```python
from build123d import *

# Parameters (mm, degrees)
BASE_FLANGE1_DEPTH = 80
CUT_EXTRUDE1_DEPTH = 110.708705215
SKETCH8_R          = 3.5
SKETCH8_W          = 7
SKETCH8_H          = 60
CUT_EXTRUDE2_DEPTH = 111.072703247
CHAMFER1_SIZE      = 2


# Sheet-metal steps are written as plain solids
with BuildPart() as part:
    # Sketch1 → Base-Flange1 (new, symmetric)
    with BuildSketch(Plane(origin=(0, 0, 0), x_dir=(0, 0, -1), z_dir=(1, 0, 0))):
        with BuildLine():
            Line((0, 50), (0, 8))
            ThreePointArc((0, 8), (2.343145751, 2.343145751), (8, 0))
            Line((8, 0), (60, 0))
            Line((60, 0), (60, 4))
            Line((60, 4), (8, 4))
            ThreePointArc((8, 4), (5.171572875, 5.171572875), (4, 8))
            Line((4, 8), (4, 50))
            Line((4, 50), (0, 50))
        make_face()
    extrude(amount=BASE_FLANGE1_DEPTH, both=True)

    # Sketch7 → Cut-Extrude1 (cut, through all)
    with BuildSketch(Plane(origin=(0, 0, -4), x_dir=(-1, 0, 0), z_dir=(0, 0, -1))):
        with BuildLine():
            Line((2.75, 50), (-2.75, 50))
            Line((-2.75, 50), (-2.75, 25))
            ThreePointArc((-2.75, 25), (0, 27.75), (2.75, 25))
            Line((2.75, 25), (2.75, 50))
        make_face()
        with BuildLine():
            ThreePointArc((2.75, 25), (0, 27.75), (-2.75, 25))
            Line((-2.75, 25), (2.75, 25))
        make_face()
        with BuildLine():
            Line((2.75, 25), (-2.75, 25))
            ThreePointArc((-2.75, 25), (0, 22.25), (2.75, 25))
        make_face()
        Polygon((-80, 30), (-25, 50), (-80, 50), align=None)
        Polygon((80, 50), (25, 50), (80, 30), align=None)
    extrude(amount=-CUT_EXTRUDE1_DEPTH, mode=Mode.SUBTRACT)

    # Sketch8 → Cut-Extrude2 (cut, through all)
    with BuildSketch(Plane(origin=(0, 4, 0), x_dir=(1, 0, 0), z_dir=(0, 1, 0))):
        with Locations((-55, 30)):
            Circle(SKETCH8_R)
        with Locations((55, 30)):
            Circle(SKETCH8_R)
        with Locations((-55, 60)):
            Rectangle(SKETCH8_W, SKETCH8_H)
        with Locations((55, 60)):
            Rectangle(SKETCH8_W, SKETCH8_H)
    extrude(amount=-CUT_EXTRUDE2_DEPTH, mode=Mode.SUBTRACT)

    # Chamfer1
    chamfer1_edges = [part.edges().sort_by_distance(p)[0] for p in [
        (80, 2, -60),
        (-80, 2, -60),
    ]]
    chamfer(chamfer1_edges, length=CHAMFER1_SIZE)


solid = part.part
```
Can you work these out from the model? Positions are in its coordinate system, mm. A direction names the side the tool comes from. Round coordinates to 2 decimals unless told otherwise and drop trailing zeros. Order: outer loops, then holes, each group sorted by start corner. A loop starts at its lowest first (then second) coordinate and runs counter-clockwise, first axis right, second up. Notation, with made-up numbers: (75.25, -17.5) -> (98.25, -17.5) arc R22 ccw to (98.25, 11.5) -> close; hole circle Ø4 at (-12.5, -14.75). An arc over 180 degrees is marked (long way). Return JSON: item names as keys, results as strings. Group by question number.
1. Will these pins go through, and if not, where does the flat tip stop? pin 1 (12.5 mm diameter, centred on x = -4.5, y = 32.5, fed in from -Z); pin 2 (5 mm diameter, centred on x = -28.5, z = -7.5, fed in from -Y); pin 3 (5 mm diameter, centred on y = 14.5, z = -7.5, fed in from -X); pin 4 (1.5 mm diameter, centred on x = -28, z = -9.5, fed in from +Y).
2. If we section it at A-A, the plane z = -40.5: Write out the boundary of the cut face in (x, y), then the cut area to 3 significant figures.
3. I need wall thicknesses on line 1 (Z direction, x = 37, y = 30); line 2 (Y direction, x = -62, z = -29.5); line 3 (Z direction, x = -59.5, y = 7). Which ranges of each line are inside material? Lowest first, please. Write a range as [from, to].
4. Which directions (+Z, -Z, +X, -X, +Y, -Y) give clear straight access to the entire face, cutting with the end or side of a thin tool? Please do faces 1 (the face through (-51.5, 2, -45)), 2 (the face through (1.12, 2.406, -2.281)), 3 (the face through (-2.75, 37, -2)), 4 (the face through (1, 4, -34)), 5 (the face through (68, 2, -60)).
5. We'd pull the mould along X, two halves only. Please class faces 6 (the face through (-68, 2, -60)), 7 (the face through (2.75, 38, -2)), 8 (the face through (52.88, 39.86, -2.03)): released by +X, released by -X, zero draft, split by the parting line, or undercut.
6. If we section it at C-C, the plane x = 69: Write out the boundary of the cut face in (y, z).
7. If we section it at B-B, the plane y = 34: Write out the boundary of the cut face in (x, z), then the cut area to 3 significant figures.
8. If we section it at D-D, the plane y = 43: Write out the boundary of the cut face in (x, z), then the cut area to 3 significant figures.
Output values:
{
 "1": {"pin 1": "z = -4", "pin 2": "y = 0", "pin 3": "through", "pin 4": "y = 4"},
 "2": {"outline": "(-80, 0) -> (-58.5, 0) -> (-58.5, 4) -> (-80, 4) -> close; (-51.5, 0) -> (51.5, 0) -> (51.5, 4) -> (-51.5, 4) -> close; (58.5, 0) -> (80, 0) -> (80, 4) -> (58.5, 4) -> close", "area": "584 mm²"},
 "3": {"line 1": "[-4, 0]", "line 2": "[0, 4]", "line 3": "[-4.13, -0.06]"},
 "4": {"face 1": "-Z, +Y, -Y", "face 2": "+Z, +X, -X, -Y", "face 3": "+Z, -Z, +Y", "face 4": "-Z, +X, -X, +Y", "face 5": "-Z, +X, -X, +Y, -Y"},
 "5": {"face 6": "zero draft", "face 7": "undercut", "face 8": "released by +X"},
 "6": {"outline": "(0, -60) -> (4, -60) -> (4, -8) arc R4 cw to (8, -4) -> (34, -4) -> (34, 0) -> (8, 0) arc R8 ccw to (0, -8) -> close"},
 "7": {"outline": "(-69, -4) -> (-2.75, -4) -> (-2.75, 0) -> (-69, 0) -> close; (2.75, -4) -> (69, -4) -> (69, 0) -> (2.75, 0) -> close", "area": "530 mm²"},
 "8": {"outline": "(-44.25, -4) -> (-2.75, -4) -> (-2.75, 0) -> (-44.25, 0) -> close; (2.75, -4) -> (44.25, -4) -> (44.25, 0) -> (2.75, 0) -> close", "area": "332 mm²"}
}
